Check sheet for the modelled part. Datum: model origin and axes. Units: mm. Give positions to 0.01 mm unless a question says otherwise; leave off trailing zeros. Write each loop counter-clockwise with the first axis right and the second up, starting at its lowest first coordinate (ties: lowest second). Pieces come first, ordered by that corner, then holes. Notation, with made-up numbers: (7, -3.75) -> (22, -3.75) arc R19 cw to (22, 25.25) -> close; hole circle Ø7 at (-24.5, 84). An arc over 180 degrees is marked (long way). Use a Markdown table: item, result. Add a question column.
1. Gauge pin test, flat ends, axial feed: P1, Ø3.5, axis at y = -139.12, z = 35, coming from the -X side; P2, Ø4.5, axis at x = 4.76, z = 206.45, coming from the -Y side; P3, Ø4.5, axis at x = 4.76, y = 105.79, coming from the +Z side (3 decimals). Record the tip position at first contact, or that the pin passes through.
2. Cross-section at B-B (z = -113.5). Enter the section's corners in (x, y) (3 decimals), then the cut area to 3 significant figures.
3. Cross-section at A-A (y = -50). Enter the section's corners in (x, z) (3 decimals), then the cut area to 3 significant figures.
4. Scan lines: probe 1 along Y at (x, z) = (6.5, -190); probe 2 along Y at (x, z) = (4.75, 35); probe 3 along Y at (x, z) = (1, 98.5). Record each from-to range of solid material in increasing order. Write a range as [from, to].
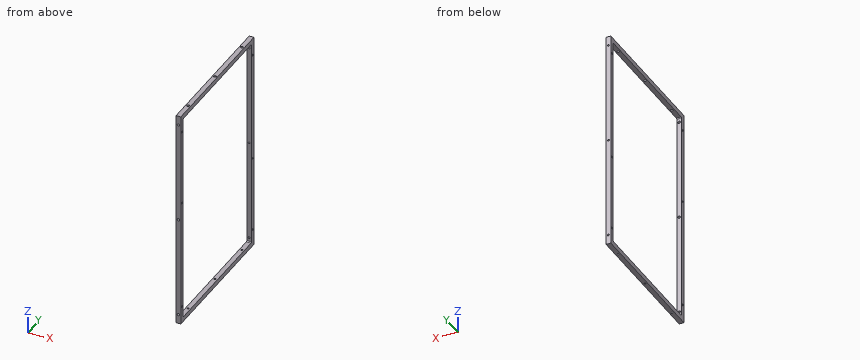
from build123d import *

# Parameters (mm, degrees)
SKETCH1_W                   = 451
SKETCH1_H                   = 287.7714167
SKETCH1_W_2                 = 431.95
SKETCH1_H_2                 = 268.7214167
EXTRUDE_THIN1_DEPTH         = 9.525
FILLET1_R                   = 2
F_10_CLEARANCE_HOLE1_D      = 4.9784
F_10_CLEARANCE_HOLE1_DEPTH  = 9.525
F_10_24_TAPPED_HOLE1_D      = 3.7973
F_10_24_TAPPED_HOLE1_DEPTH  = 14.95
F_10_24_TAPPED_HOLE1_TIP    = 1.140824014
F_10_CLEARANCE_HOLE2_D      = 5.1054
F_10_CLEARANCE_HOLE2_DEPTH  = 20
F_10_CLEARANCE_HOLE2_TIP    = 1.533816902
F_10_24_TAPPED_HOLE2_SIDE_D = 3.7973
F_10_24_TAPPED_HOLE2_D      = 3.7973
F_10_24_TAPPED_HOLE2_DEPTH  = 14.95
F_10_24_TAPPED_HOLE2_TIP    = 1.140824014


with BuildPart() as part:
    # Sketch1 → Extrude-Thin1 (new body)
    with BuildSketch(Plane(origin=(0, 0, 0), x_dir=(0, 0, -1), z_dir=(1, 0, 0))):
        Rectangle(SKETCH1_W, SKETCH1_H)
        Rectangle(SKETCH1_W_2, SKETCH1_H_2, mode=Mode.SUBTRACT)
    extrude(amount=EXTRUDE_THIN1_DEPTH)

    # Fillet1
    fillet1_edges = [part.edges().sort_by_distance(p)[0] for p in [
        (4.7625, 134.36070835, 215.975),
        (4.7625, -134.36070835, 215.975),
        (4.7625, -134.36070835, -215.975),
        (4.7625, 134.36070835, -215.975),
    ]]
    fillet(fillet1_edges, radius=FILLET1_R)

    # #10 Clearance Hole1
    with Locations(Plane(origin=(0, -143.88570835, 0), x_dir=(-1, 0, 0), z_dir=(0, -1, 0))):
        with Locations((-4.7625, 206.45), (-4.7625, 0), (-4.7625, -206.45)):
            Hole(F_10_CLEARANCE_HOLE1_D / 2, depth=F_10_CLEARANCE_HOLE1_DEPTH)

    # #10-24 Tapped Hole1
    with Locations(Plane(origin=(0, 0, -225.5), x_dir=(-1, 0, 0), z_dir=(0, 0, -1))):
        with Locations((-4.7625, 105.78570835), (-4.7625, 0), (-4.7625, -105.78570835)):
            Hole(F_10_24_TAPPED_HOLE1_D / 2, depth=F_10_24_TAPPED_HOLE1_DEPTH)
            with Locations((0, 0, -(F_10_24_TAPPED_HOLE1_DEPTH + F_10_24_TAPPED_HOLE1_TIP / 2))):  # 118° drill point
                Cone(0, F_10_24_TAPPED_HOLE1_D / 2, F_10_24_TAPPED_HOLE1_TIP, mode=Mode.SUBTRACT)

    # #10 Clearance Hole2
    with Locations(Plane.XY.offset(225.5)):
        with Locations((4.7625, 105.78570835), (4.7625, 0), (4.7625, -105.78570835)):
            Hole(F_10_CLEARANCE_HOLE2_D / 2, depth=F_10_CLEARANCE_HOLE2_DEPTH)
            with Locations((0, 0, -(F_10_CLEARANCE_HOLE2_DEPTH + F_10_CLEARANCE_HOLE2_TIP / 2))):  # 118° drill point
                Cone(0, F_10_CLEARANCE_HOLE2_D / 2, F_10_CLEARANCE_HOLE2_TIP, mode=Mode.SUBTRACT)

    # #10-24 Tapped Hole2 side (through all)
    with Locations(Plane.ZY):
        with Locations((-190, 139.12320835), (-35, 139.12320835), (-190, -139.12320835), (35, -139.12320835), (190, -139.12320835), (190, 139.12320835)):
            Hole(F_10_24_TAPPED_HOLE2_SIDE_D / 2)

    # #10-24 Tapped Hole2
    with Locations(Plane(origin=(0, 143.88570835, 0), x_dir=(1, 0, 0), z_dir=(0, 1, 0))):
        with Locations((4.7625, 206.45), (4.7625, 0), (4.7625, -206.45)):
            Hole(F_10_24_TAPPED_HOLE2_D / 2, depth=F_10_24_TAPPED_HOLE2_DEPTH)
            with Locations((0, 0, -(F_10_24_TAPPED_HOLE2_DEPTH + F_10_24_TAPPED_HOLE2_TIP / 2))):  # 118° drill point
                Cone(0, F_10_24_TAPPED_HOLE2_D / 2, F_10_24_TAPPED_HOLE2_TIP, mode=Mode.SUBTRACT)


solid = part.part
Worked answers:
| question | item | result |
|---|---|---|
| 1 | P1 | passes through |
| 1 | P2 | stops at y = 134.36 |
| 1 | P3 | stops at z = -215.975 |
| 2 | outline | (0, -143.886) -> (9.525, -143.886) -> (9.525, -134.361) -> (0, -134.361) -> close; (0, 134.361) -> (9.525, 134.361) -> (9.525, 143.886) -> (0, 143.886) -> close |
| 2 | area | 181 mm² |
| 3 | outline | (0, -225.5) -> (9.525, -225.5) -> (9.525, -215.975) -> (0, -215.975) -> close; (0, 215.975) -> (9.525, 215.975) -> (9.525, 225.5) -> (0, 225.5) -> close |
| 3 | area | 181 mm² |
| 4 | probe 1 | y = [-143.89, -141.02], [-137.22, -134.36], [134.36, 137.22], [141.02, 143.89] |
| 4 | probe 2 | y = [-143.89, -141.02], [-137.22, -134.36], [134.36, 143.89] |
| 4 | probe 3 | y = [-143.89, -134.36], [134.36, 143.89] |
